The drawing under review shows one solid part. Ordinate dimensions are in mm from its lowest x, y, z. Round coordinates to 2 decimals unless told otherwise and drop trailing zeros. Write each loop counter-clockwise with the first axis right and the second up, starting at its lowest first coordinate (ties: lowest second). Pieces come first, ordered by that corner, then holes. Notation, with made-up numbers: M 49,50 L 56,50 A26 cw 56,87 Z; hole C 32.5,77.5 d10. An arc over 180 degrees is marked long. One line per item, written item: value. Start each with the question number.
1) Wall thickness on probe 1 along Z at (x, y) = (35.5, 0.9); probe 2 along X at (y, z) = (0.9, 65); probe 3 along Z at (x, y) = (18, 0.95): over which ranges is each line inside the solid? List them lowest first.
2) Take a section at B-B, the plane x = 41.5. Write out the cut boundary in (y, z).
3) Take a section at C-C, the plane y = 1.15. Write out the cut boundary in (x, z), and give its area (3 significant figures).
4) Take a section at A-A, the plane z = 19. Write out the cut boundary in (x, y).
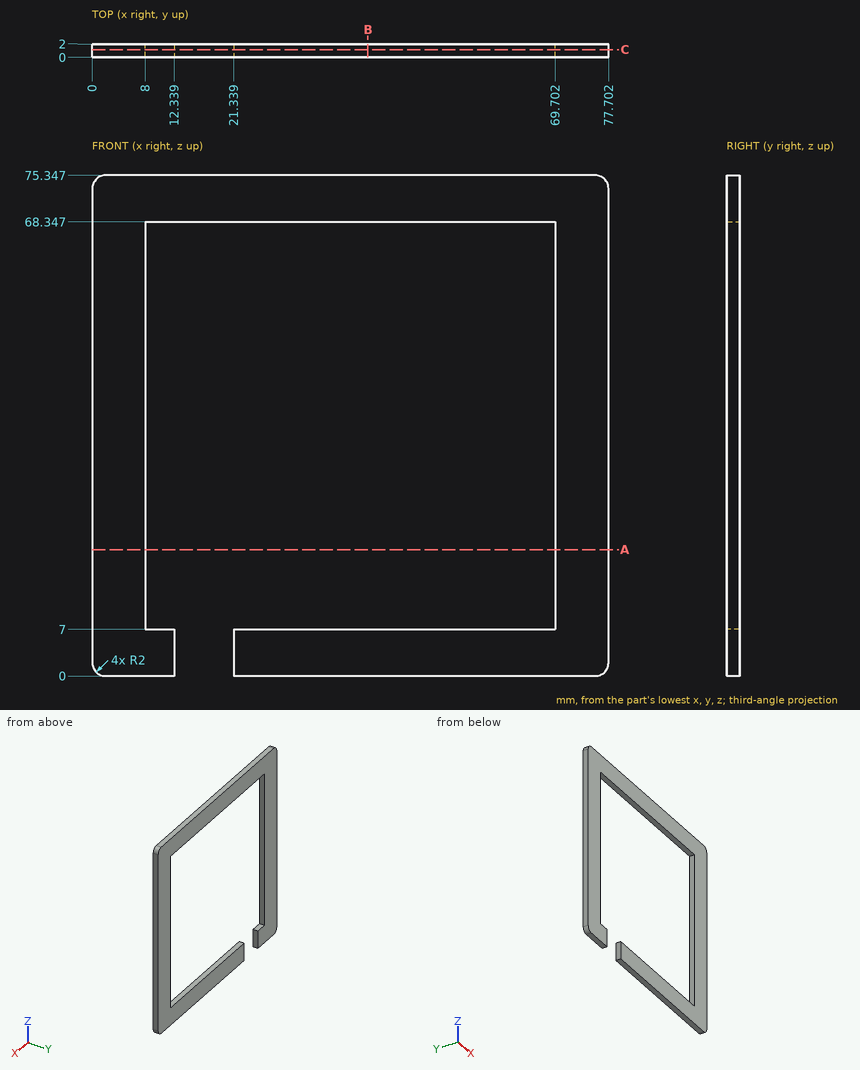
Checked values:
1. probe 1: z = 0 to 7, 68.35 to 75.35
1. probe 2: x = 0 to 8, 69.7 to 77.7
1. probe 3: z = 68.35 to 75.35
2. outline: M 0,0 L 2,0 L 2,7 L 0,7 Z; M 0,68.35 L 2,68.35 L 2,75.35 L 0,75.35 Z
3. outline: M 0,2 A2 ccw 2,0 L 12.34,0 L 12.34,7 L 8,7 L 8,68.35 L 69.7,68.35 L 69.7,7 L 21.34,7 L 21.34,0 L 75.7,0 A2 ccw 77.7,2 L 77.7,73.35 A2 ccw 75.7,75.35 L 2,75.35 A2 ccw 0,73.35 Z
3. area: 2,000 mm2
4. outline: M 0,0 L 8,0 L 8,2 L 0,2 Z; M 69.7,0 L 77.7,0 L 77.7,2 L 69.7,2 Z
